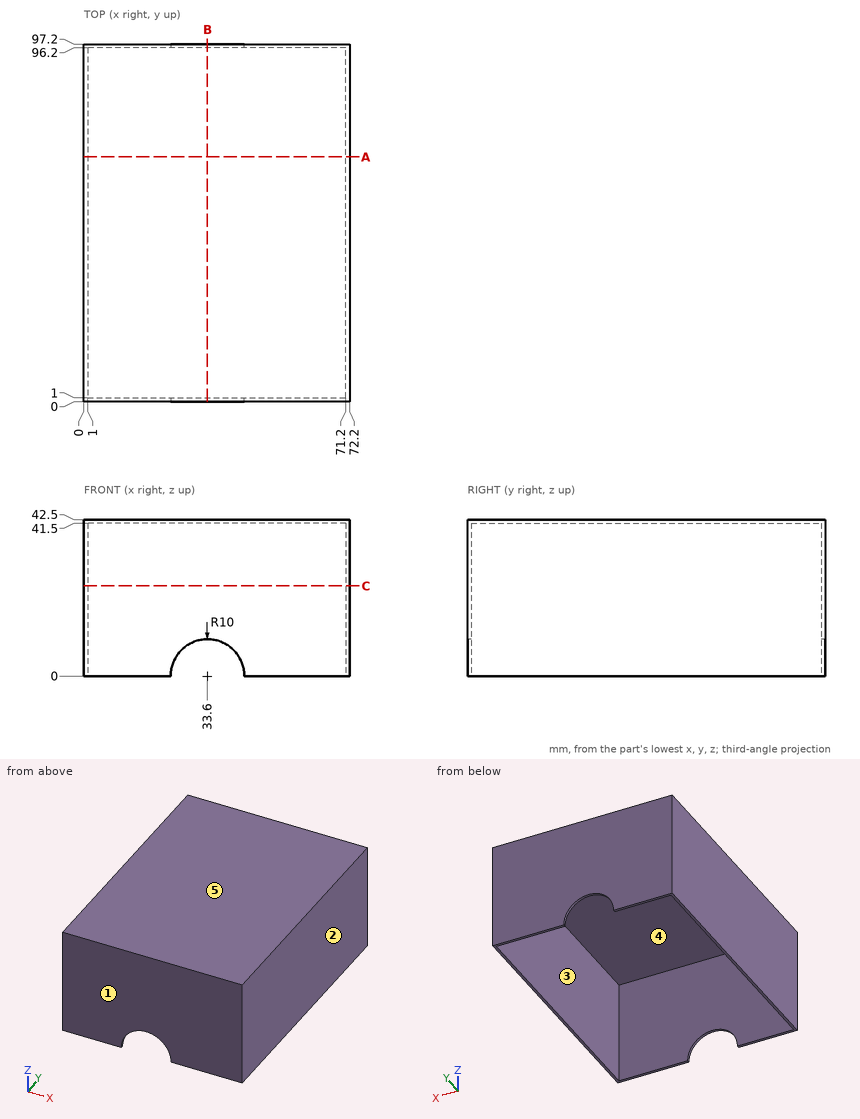
Source: three-view drawing plus pictorial views. Frame: mm from the lowest corner of the part. A direction names the side the tool comes from. Give positions to 0.01 mm unless a question says otherwise; leave off trailing zeros. Write each loop counter-clockwise with the first axis right and the second up, starting at its lowest first coordinate (ties: lowest second). Pieces come first, ordered by that corner, then holes. Notation, with made-up numbers: (3, 65.5) - (46, 65.5) arc R12 ccw to (46, 77.5) - close; hole circle Ø7 at (49, -8). An arc over 180 degrees is marked (long way). Write item = value, one per line. Start each with the question number.
1. Ray query, L1, parallel to Y at x = 41.5, z = 19.5; L2, parallel to X at y = 24.5, z = 26.5; L3, parallel to Z at x = 25, y = 34.5. Return the intervals inside material, ascending.
2. Section query C-C, the plane z = 24.5. Output: boundary loops of the cut face in (x, y), then the cut area to 3 significant figures.
3. First-contact query: pin 1 Ø4 at (x, y) = (53.5, 79.5) entering from -Z. Flat tip, straight axial feed; report the tip coordinate or a pass-through.
4. Section query B-B, the plane x = 33.6. Output: boundary loops of the cut face in (y, z), then the cut area to 3 significant figures.
5. Section query A-A, the plane y = 66.5. Output: boundary loops of the cut face in (x, z).
6. Access query for the marked faces 4 and 5. Directions: +Z, -Z, +X, -X, +Y, -Y. A direction counts if a zero-diameter tool reaches every point of the face in a straight line with its end or side. Return the directions, or none.
7. Mould query, pull axis X, two halves, no side actions, for the marked faces 1, 2 and 3. Classes: released by +X, released by -X, zero draft, split by the parting line, or undercut.
Check sheet entries:
q1.L1 = 0 to 1, 96.2 to 97.2
q1.L2 = 0 to 1, 71.2 to 72.2
q1.L3 = 41.5 to 42.5
q2.outline = (0, 0) - (72.2, 0) - (72.2, 97.2) - (0, 97.2) - close; hole (1, 1) - (71.2, 1) - (71.2, 96.2) - (1, 96.2) - close
q2.area = 335 mm2
q3.pin_1 = 41.5
q4.outline = (0, 10) - (1, 10) - (1, 41.5) - (96.2, 41.5) - (96.2, 10) - (97.2, 10) - (97.2, 42.5) - (0, 42.5) - close
q4.area = 160 mm2
q5.outline = (0, 0) - (1, 0) - (1, 41.5) - (71.2, 41.5) - (71.2, 0) - (72.2, 0) - (72.2, 42.5) - (0, 42.5) - close
q6.face_4 = -Z
q6.face_5 = +Z, +X, -X, +Y, -Y
q7.face_1 = zero draft
q7.face_2 = released by +X
q7.face_3 = undercut
